The model under review builds one solid part; all positions refer to its coordinate system, in mm. Face numbers are marked on the shaded views. A direction names the side the tool comes from. Coordinates: 2 decimals unless noted, no trailing zeros. Loops run counter-clockwise (first coordinate to the right, second up) from the corner with the lowest first, then second, coordinate; pieces in that order, holes last. Notation, with made-up numbers: M 35,26 L 89,26 A29 cw 89,46 Z; hole C -26.75,72.25 d1. An arc over 180 degrees is marked long. Use CSV: the item, a comma, the result in double quotes. Start each with the question number.
from build123d import *

# Parameters (mm, degrees)
PAD_DEPTH            = 9
SKETCH001_W          = 37.346859
SKETCH001_H          = 35.838272
POCKET_DEPTH         = 6
POCKET_DEPTH_BACK    = 100
SKETCH002_R          = 2.5
POCKET001_DEPTH      = 38.001
SKETCH003_R          = 2.5
POCKET002_DEPTH      = 38.001
SKETCH004_W          = 20
SKETCH004_H          = 20
POCKET003_DEPTH      = 9.001
POCKET003_DEPTH_BACK = 9.001


with BuildPart() as part:
    # Sketch → Pad (new body, symmetric)
    with BuildSketch(Plane.XY):
        Polygon((0, 0), (0, 38), (5, 38), (38, 5), (38, 0), align=None)
    extrude(amount=PAD_DEPTH, both=True)

    # Sketch001 → Pocket (cut, two sides)
    with BuildSketch(Plane.XY) as pocket_sk:
        with Locations((23.673429, 22.919136)):
            Rectangle(SKETCH001_W, SKETCH001_H)
    extrude(amount=-POCKET_DEPTH, mode=Mode.SUBTRACT)
    extrude(pocket_sk.sketch, amount=POCKET_DEPTH_BACK, mode=Mode.SUBTRACT)

    # Sketch002 (on Face2 of Pocket) → Pocket001 (cut, through all)
    with BuildSketch(Plane.XZ):
        with Locations((15, 0)):
            Circle(SKETCH002_R)
        with Locations((30, 0)):
            Circle(SKETCH002_R)
    extrude(amount=-POCKET001_DEPTH, mode=Mode.SUBTRACT)

    # Sketch003 (on Face1 of Pocket001) → Pocket002 (cut, through all)
    with BuildSketch(Plane(origin=(0, 0, 0), x_dir=(0, -1, 0), z_dir=(-1, 0, 0))):
        with Locations((-30, 0)):
            Circle(SKETCH003_R)
        with Locations((-15, 0)):
            Circle(SKETCH003_R)
    extrude(amount=-POCKET002_DEPTH, mode=Mode.SUBTRACT)

    # Sketch004 → Pocket003 (cut, two sides)
    with BuildSketch(Plane.XY) as pocket003_sk:
        with Locations((30, 15)):
            Rectangle(SKETCH004_W, SKETCH004_H)
    extrude(amount=-POCKET003_DEPTH, mode=Mode.SUBTRACT)
    extrude(pocket003_sk.sketch, amount=POCKET003_DEPTH_BACK, mode=Mode.SUBTRACT)


solid = part.part
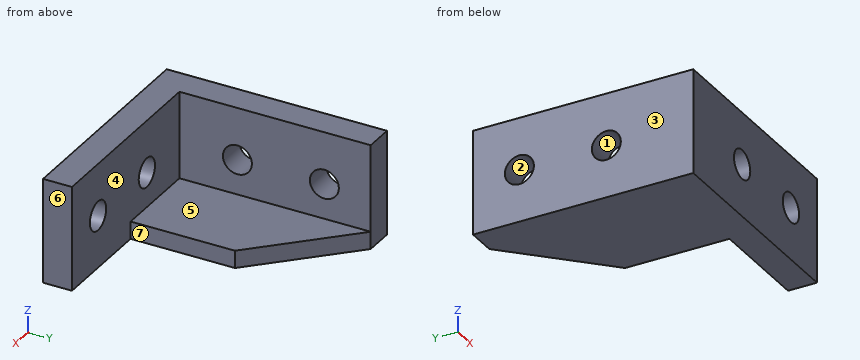
1. Add section B-B (x = 30). Write out the cut boundary in (y, z).
2. To check wall thickness, follow line 1 along Z through (x, y) = (1.15, 30); line 2 along X through (y, z) = (4, -1.75); line 3 along Y through (x, z) = (20, 8). State the ranges of each line that lie inside material, in increasing order.
3. For the marked faces 5, 6 and 7, list the 3-axis set-ups (+Z, -Z, +X, -X, +Y, -Y) from which the entire face can be reached by the end or side of a thin tool; tool diameter is ignored.
4. Add section D-D (z = 0). Write out the cut boundary in (x, y).
5. Draft analysis for pull direction Y (two halves, no side actions). For the marked faces 1, 2, 3 and 4, state which applies: released by +Y, released by -Y, zero draft, split by the parting line, or undercut.
6. Add section C-C (z = -7.5). Write out the cut boundary in (x, y), plus the area to 4 significant figures.
7. Add section A-A (y = 15). Write out the cut boundary in (x, z).
8. Insertion check: pin 1 Ø1 at (y, z) = (26, -1.5) entering from +X; pin 2 Ø4 at (x, z) = (30, 0) entering from -Y; pin 3 Ø5.5 at (x, z) = (14, 3) entering from +Y; pin 4 Ø4.5 at (x, y) = (10.5, 16) entering from +Z. Each pin has a flat end and moves straight along its axis. Give the tip position at first contact, or say it passes through.
Solved:
1,outline,"M 0,-9 L 5,-9 L 5,-2.5 L 0,-2.5 Z; M 0,2.5 L 5,2.5 L 5,9 L 0,9 Z"
2,line 1,"z = -9 to -2.5, 2.5 to 9"
2,line 2,"x = 0 to 13.21, 16.79 to 28.21, 31.79 to 38"
2,line 3,"y = 0 to 5"
3,face 5,"+Z, +X, +Y"
3,face 6,"+Z, -Z, +X, +Y, -Y"
3,face 7,"+Z, -Z, +X, +Y"
4,outline,"M 0,0 L 12.5,0 L 12.5,5 L 5,5 L 5,12.5 L 0,12.5 Z; M 0,17.5 L 5,17.5 L 5,27.5 L 0,27.5 Z; M 0,32.5 L 5,32.5 L 5,38 L 0,38 Z; M 17.5,0 L 27.5,0 L 27.5,5 L 17.5,5 Z; M 32.5,0 L 38,0 L 38,5 L 32.5,5 Z"
5,face 1,"undercut"
5,face 2,"undercut"
5,face 3,"zero draft"
5,face 4,"released by +Y"
6,outline,"M 0,0 L 38,0 L 38,5 L 20,5 L 20,23 L 5,38 L 0,38 Z"
6,area,"737.5 mm^2"
7,outline,"M 0,-9 L 20,-9 L 20,-6 L 5,-6 L 5,-2.5 L 0,-2.5 Z; M 0,2.5 L 5,2.5 L 5,9 L 0,9 Z"
8,pin 1,"stops at x = 5"
8,pin 2,"passes through"
8,pin 3,"stops at y = 5"
8,pin 4,"stops at z = -6"
